```python
from build123d import *

# Parameters (mm, degrees)
SKETCH1_R               = 15.5
SKETCH1_R_2             = 14.75
BOSS_EXTRUDE1_DEPTH     = 300
SKETCH4_W               = 35
SKETCH4_H               = 125
BOSS_EXTRUDE2_DEPTH     = 5
CUT_EXTRUDE2_DEPTH      = 50
CUT_EXTRUDE2_DEPTH_BACK = 40
FILLET2_R               = 5


with BuildPart() as part:
    # Sketch1 → Boss-Extrude1 (new body)
    with BuildSketch(Plane(origin=(0, 0, 0), x_dir=(1, 0, 0), z_dir=(0, 1, 0))):
        with Locations(Location((0, 0, 0), (0, 0, 270))):
            Circle(SKETCH1_R)
        with Locations(Location((0, 0, 0), (0, 0, 270))):
            Circle(SKETCH1_R_2, mode=Mode.SUBTRACT)
    extrude(amount=BOSS_EXTRUDE1_DEPTH)

    # Sketch4 → Boss-Extrude2 (add)
    with BuildSketch(Plane(origin=(0, 300, 0), x_dir=(1, 0, 0), z_dir=(0, 1, 0))):
        Rectangle(SKETCH4_W, SKETCH4_H)
    extrude(amount=BOSS_EXTRUDE2_DEPTH)

    # Sketch2 → Cut-Extrude2 (cut, two sides: drawn at the far end of the back side and taken through both)
    with BuildSketch(Plane.XY.offset(-CUT_EXTRUDE2_DEPTH_BACK)):
        with BuildLine():
            Line((15.5, 33.559719433), (15.5, 259.086340433))
            ThreePointArc((15.5, 259.086340433), (8.366249541, 256.521002237), (4.5, 250))
            Line((4.5, 250), (4.5, 40))
            ThreePointArc((4.5, 40), (9.126672498, 35.288216236), (15.5, 33.559719433))
        make_face()
    extrude(amount=CUT_EXTRUDE2_DEPTH + CUT_EXTRUDE2_DEPTH_BACK, mode=Mode.SUBTRACT)

    # Fillet2
    fillet2_edges = [part.edges().sort_by_distance(p)[0] for p in [
        (0, 305, -62.5),
        (0, 305, 62.5),
        (-17.5, 305, 0),
        (17.5, 305, 0),
    ]]
    fillet(fillet2_edges, radius=FILLET2_R - 0.0001)  # a hair under: the kernel refuses the full size


solid = part.part
```
For this review, take the finished solid that the model builds, in its own axes (mm). A direction names the side the tool comes from. Coordinates: 2 decimals unless noted, no trailing zeros. Order: outer loops, then holes, each group sorted by start corner. A loop starts at its lowest first (then second) coordinate and runs counter-clockwise, first axis right, second up. Notation, with made-up numbers: (-6.75, 10) -> (37.25, 10) arc R16 ccw to (37.25, 17) -> close; hole circle Ø3 at (80.25, -28.75). An arc over 180 degrees is marked (long way). Answer as CSV lines item,"result".
Q1. We need section D-D (y = 214). State the section outline as (x, z) points.
Model answer:
outline,"(4.5, -14.83) -> (4.5, -14.05) arc R14.75 cw (long way) to (4.5, 14.05) -> (4.5, 14.83) arc R15.5 ccw (long way) to start"
Q2. Draft analysis for pull direction Z (two halves, no side actions). For faces 4 (the face through (-16.07, 303.5, -0.88)), 5 (the face through (0, 300, 0)), 6 (the face through (-13.086, 147.9, 6.806)), 7 (the face through (0.25, 303.57, -61)), state which applies: released by +Z, released by -Z, zero draft, split by the parting line, or undercut.
Model answer:
face 4,"zero draft"
face 5,"undercut"
face 6,"undercut"
face 7,"released by -Z"
Q3. Clearance check with flat-ended pins moving along their axes: pin 1 Ø0.9 at (y, z) = (122, -14.5) entering from +X; pin 2 Ø3 at (x, z) = (-13.5, 1) entering from +Y; pin 3 Ø6 at (x, z) = (-4, -33) entering from -Y; pin 4 Ø12 at (x, y) = (-8.5, 144) entering from -Z. State where each tip first meets the part, or that it passes through.
Model answer:
pin 1,"stops at x = 4.5"
pin 2,"stops at y = 305"
pin 3,"stops at y = 300"
pin 4,"stops at z = -15.3"
Q4. Wall thickness on line 1 along Z through (x, y) = (-1, 241); line 2 along X through (y, z) = (112, 0); line 3 along Y through (x, z) = (-11.5, -15.5): over which ranges is each line inside the solid? List them lowest first. Write a range as [from, to].
Model answer:
line 1,"z = [-15.47, -14.72], [14.72, 15.47]"
line 2,"x = [-15.5, -14.75]"
line 3,"y = [300, 305]"
Q5. For faces 1 (the face through (-15.13, 147.9, -3.36)), 2 (the face through (0.25, 303.57, 61)), 3 (the face through (15.25, 259.084, -0.069)), list the 3-axis set-ups (+Z, -Z, +X, -X, +Y, -Y) from which the entire face can be reached by the end or side of a thin tool; tool diameter is ignored.
Model answer:
face 1,"-Y"
face 2,"+Z, +X, -X, +Y"
face 3,"+Z, -Z, +X"
